Model file for the job. Use its own axes, mm. Face numbers are marked on the shaded views. Coordinates: 2 decimals unless noted, no trailing zeros. Order: outer loops, then holes, each group sorted by start corner. A loop starts at its lowest first (then second) coordinate and runs counter-clockwise, first axis right, second up. Notation, with made-up numbers: (-1.5, 16) -> (49.5, 16) arc R11 cw to (49.5, 22) -> close; hole circle Ø3 at (69, 8.25). An arc over 180 degrees is marked (long way). Use CSV: the item, a comma, the result in double quotes. Start each with the question number.
(1) Pin check, flat tips, straight feed: pin 1 Ø2 at (y, z) = (3, 116) entering from -X; pin 2 Ø1.9 at (x, z) = (0.5, 114.5) entering from +Y; pin 3 Ø1.6 at (y, z) = (1, 111) entering from +X. Stop position of each tip, or through.
(2) Cut at A-A on z = -25. Write the cut outline in (x, y).
(3) Probe L1, parallel to Y at x = 0, z = 99 (3 decimals); L2, parallel to Y at x = -13.5, z = -69.5; L3, parallel to Z at x = -13.5, y = -1.5. List the from-to ranges inside material, lowest first.
(4) Cut at B-B on z = -67. Write the cut outline in (x, y), plus the area to 3 significant figures.
(5) Pull direction Y, two halves, no side cores. Call the marked faces 1 and 2: pulls with the +Y half, pulls with the -Y half, needs draft (parallel to the pull), parting line crosses it, or undercut.
(6) Cut at C-C on z = 36. Write the cut outline in (x, y) (3 decimals).
```python
from build123d import *

# Parameters (mm, degrees)
PAD_DEPTH            = 25
PAD_DEPTH_BACK       = 25
PAD001_START         = 5
PAD001_DEPTH         = 115
PAD002_DEPTH         = 6
PAD002_DEPTH_BACK    = 6
POCKET_DEPTH         = 10.001
POCKET_DEPTH_BACK    = 10.001
POCKET001_DEPTH      = 120.001
PAD003_DEPTH         = 2
LINEARPATTERN_COUNT  = 2
LINEARPATTERN_PITCH  = 8
SKETCH006_W          = 15
SKETCH006_H          = 1
POCKET002_DEPTH      = 7
PAD004_DEPTH         = 6
PAD004_DEPTH_BACK    = 6
SKETCH008_W          = 3.8
SKETCH008_H          = 20
POCKET003_DEPTH      = 60.001
POCKET003_DEPTH_BACK = 60.001
POCKET004_DEPTH      = 10.001
POCKET004_DEPTH_BACK = 10.001
FILLET_R             = 10
FILLET001_R          = 10
FILLET002_R          = 5
FILLET003_R          = 10
FILLET004_R          = 1
FILLET005_R          = 1
SKETCH010_W          = 10
SKETCH010_H          = 30
POCKET005_DEPTH      = 60.001
POCKET005_DEPTH_BACK = 60.001
SKETCH011_W          = 10
SKETCH011_H          = 30
POCKET006_DEPTH      = 60.001
POCKET006_DEPTH_BACK = 60.001
FILLET006_R          = 10
CHAMFER_SIZE         = 1
CHAMFER001_SIZE      = 1


with BuildPart() as part:
    # Sketch → Pad (new body, two sides)
    with BuildSketch(Plane.YZ) as pad_sk:
        Polygon((10, -4.142136), (10, 4.142136), (4.142136, 10), (-4.142136, 10), (-10, 4.142136), (-10, -4.142136), (-4.142136, -10), (4.142136, -10), align=None)
        Polygon((2.5, 1.035534), (1.035534, 2.5), (-1.035534, 2.5), (-2.5, 1.035534), (-2.5, -1.035534), (-1.035534, -2.5), (1.035534, -2.5), (2.5, -1.035534), align=None, mode=Mode.SUBTRACT)
    extrude(amount=PAD_DEPTH)
    extrude(pad_sk.sketch, amount=-PAD_DEPTH_BACK)

    # Sketch001 → Pad001 (join)
    with BuildSketch(Plane.XY.offset(PAD001_START)):
        Polygon((4.5, -1.863961), (4.5, 1.863961), (1.863961, 4.5), (-1.863961, 4.5), (-4.5, 1.863961), (-4.5, -1.863961), (-1.863961, -4.5), (1.863961, -4.5), align=None)
        Polygon((1.575, -0.652386), (1.575, 0.652386), (0.652386, 1.575), (-0.652386, 1.575), (-1.575, 0.652386), (-1.575, -0.652386), (-0.652386, -1.575), (0.652386, -1.575), align=None, mode=Mode.SUBTRACT)
    extrude(amount=PAD001_DEPTH)

    # Sketch002 → Pad002 (join, two sides)
    with BuildSketch(Plane.XZ) as pad002_sk:
        Polygon((-25, 8), (25, 8), (25, 13), (10, 42), (10, 47), (13, 47), (13, 50), (-13, 50), (-13, 47), (-10, 47), (-10, 42), (-25, 13), align=None)
    extrude(amount=PAD002_DEPTH)
    extrude(pad002_sk.sketch, amount=-PAD002_DEPTH_BACK)

    # Sketch003 → Pocket (cut, two sides)
    with BuildSketch(Plane.XZ) as pocket_sk:
        with BuildLine():
            ThreePointArc((7, 8), (0, 15), (-7, 8))
            Line((-7, 8), (7, 8))
        make_face()
    extrude(amount=-POCKET_DEPTH, mode=Mode.SUBTRACT)
    extrude(pocket_sk.sketch, amount=POCKET_DEPTH_BACK, mode=Mode.SUBTRACT)

    # Sketch004 → Pocket001 (cut, through all)
    with BuildSketch(Plane.XY):
        Polygon((1.575, -0.652386), (1.575, 0.652386), (0.652386, 1.575), (-0.652386, 1.575), (-1.575, 0.652386), (-1.575, -0.652386), (-0.652386, -1.575), (0.652386, -1.575), align=None)
    extrude(amount=POCKET001_DEPTH, mode=Mode.SUBTRACT)

    # Sketch005 (on Face68 of Pocket001) → Pad003 (join)
    with BuildSketch(Plane(origin=(0, 0, 120), x_dir=(0, -1, 0), z_dir=(0, 0, 1))):
        Polygon((5.543277, -2.296101), (5.543277, 2.296101), (2.296101, 5.543277), (-2.296101, 5.543277), (-5.543277, 2.296101), (-5.543277, -2.296101), (-2.296101, -5.543277), (2.296101, -5.543277), align=None)
        Polygon((1.339392, -3.233578), (3.233578, -1.339392), (3.233578, 1.339392), (1.339392, 3.233578), (-1.339392, 3.233578), (-3.233578, 1.339392), (-3.233578, -1.339392), (-1.339392, -3.233578), align=None, mode=Mode.SUBTRACT)
    pad003 = extrude(amount=-PAD003_DEPTH)

    # LinearPattern: Pad003 ×2
    with Locations(*[(0, 0, -i * LINEARPATTERN_PITCH) for i in range(1, LINEARPATTERN_COUNT)]):
        add(pad003)

    # Sketch006 (on Face80 of LinearPattern) → Pocket002 (cut)
    with BuildSketch(Plane(origin=(0, 0, 120), x_dir=(0, -1, 0), z_dir=(0, 0, 1))):
        Rectangle(SKETCH006_W, SKETCH006_H)
    extrude(amount=-POCKET002_DEPTH, mode=Mode.SUBTRACT)

    # Sketch007 → Pad004 (join, two sides)
    with BuildSketch(Plane.XZ) as pad004_sk:
        Polygon((-25, -5), (25, -5), (25, -15), (60, -50), (60, -80), (-60, -80), (-60, -50), (-25, -15), align=None)
    extrude(amount=PAD004_DEPTH)
    extrude(pad004_sk.sketch, amount=-PAD004_DEPTH_BACK)

    # Sketch008 → Pocket003 (cut, two sides)
    with BuildSketch(Plane.YZ) as pocket003_sk:
        with Locations((0, -71)):
            Rectangle(SKETCH008_W, SKETCH008_H)
    extrude(amount=-POCKET003_DEPTH, mode=Mode.SUBTRACT)
    extrude(pocket003_sk.sketch, amount=POCKET003_DEPTH_BACK, mode=Mode.SUBTRACT)

    # Sketch009 → Pocket004 (cut, two sides)
    with BuildSketch(Plane.XZ) as pocket004_sk:
        Polygon((-5.142136, -8.142136), (5.142136, -8.142136), (45, -48), (45, -56), (-45, -56), (-45, -48), align=None)
    extrude(amount=-POCKET004_DEPTH, mode=Mode.SUBTRACT)
    extrude(pocket004_sk.sketch, amount=POCKET004_DEPTH_BACK, mode=Mode.SUBTRACT)

    # Fillet
    fillet_edges = [part.edges().sort_by_distance(p)[0] for p in [
        (25, 0, -15),
        (-25, 0, -15),
    ]]
    fillet(fillet_edges, radius=FILLET_R)

    # Fillet001
    fillet001_edges = [part.edges().sort_by_distance(p)[0] for p in [
        (-60, 0, -50),
        (60, 0, -50),
    ]]
    fillet(fillet001_edges, radius=FILLET001_R)

    # Fillet002
    fillet002_edges = [part.edges().sort_by_distance(p)[0] for p in [
        (-45, 0, -56),
        (-45, 0, -48),
        (45, 0, -48),
        (45, 0, -56),
    ]]
    fillet(fillet002_edges, radius=FILLET002_R)

    # Fillet003
    fillet003_edges = [part.edges().sort_by_distance(p)[0] for p in [
        (-25, 0, 13),
        (-10, 0, 42),
        (10, 0, 42),
        (25, 0, 13),
    ]]
    fillet(fillet003_edges, radius=FILLET003_R)

    # Fillet004
    fillet004_edges = [part.edges().sort_by_distance(p)[0] for p in [
        (10, 0, 47),
        (13, 0, 47),
        (13, 0, 50),
    ]]
    fillet(fillet004_edges, radius=FILLET004_R)

    # Fillet005
    fillet005_edges = [part.edges().sort_by_distance(p)[0] for p in [
        (-10, 0, 47),
        (-13, 0, 47),
        (-13, 0, 50),
    ]]
    fillet(fillet005_edges, radius=FILLET005_R)

    # Sketch010 → Pocket005 (cut, two sides)
    with BuildSketch(Plane.YZ) as pocket005_sk:
        with Locations((11, 0)):
            Rectangle(SKETCH010_W, SKETCH010_H)
    extrude(amount=-POCKET005_DEPTH, mode=Mode.SUBTRACT)
    extrude(pocket005_sk.sketch, amount=POCKET005_DEPTH_BACK, mode=Mode.SUBTRACT)

    # Sketch011 → Pocket006 (cut, two sides)
    with BuildSketch(Plane.YZ) as pocket006_sk:
        with Locations((-11, 0)):
            Rectangle(SKETCH011_W, SKETCH011_H)
    extrude(amount=-POCKET006_DEPTH, mode=Mode.SUBTRACT)
    extrude(pocket006_sk.sketch, amount=POCKET006_DEPTH_BACK, mode=Mode.SUBTRACT)

    # Fillet006
    fillet006_edges = [part.edges().sort_by_distance(p)[0] for p in [
        (60, -3.95, -80),
        (60, 3.95, -80),
        (-60, -3.95, -80),
        (-60, 3.95, -80),
    ]]
    fillet(fillet006_edges, radius=FILLET006_R)

    # Chamfer
    chamfer_edges = [part.edges().sort_by_distance(p)[0] for p in [
        (1.39805, 5.543277, 120),
        (3.919689, 3.919689, 120),
        (5.543277, 0, 120),
        (3.919689, -3.919689, 120),
        (1.39805, -5.543277, 120),
    ]]
    chamfer(chamfer_edges, length=CHAMFER_SIZE)

    # Chamfer001
    chamfer001_edges = [part.edges().sort_by_distance(p)[0] for p in [
        (-1.39805, 5.543277, 120),
        (-3.919689, 3.919689, 120),
        (-5.543277, 0, 120),
        (-3.919689, -3.919689, 120),
        (-1.39805, -5.543277, 120),
    ]]
    chamfer(chamfer001_edges, length=CHAMFER001_SIZE)


solid = part.part
```
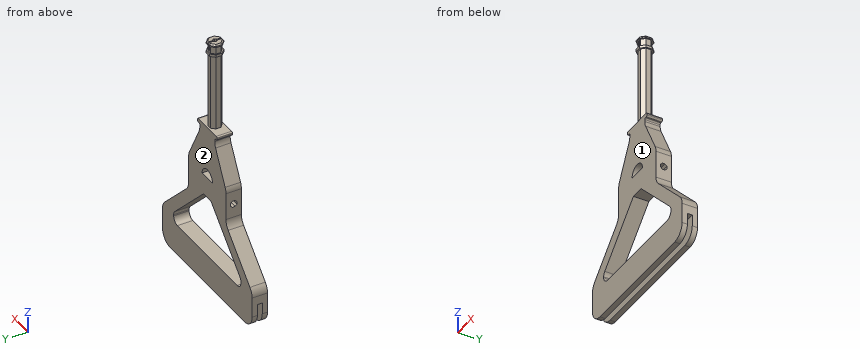
Outcome:
1,pin 1,"x = -4.36"
1,pin 2,"y = 4.5"
1,pin 3,"x = 5.54"
2,outline,"(-35, -6) -> (-22, -6) -> (-22, 6) -> (-35, 6) -> close; (22, -6) -> (35, -6) -> (35, 6) -> (22, 6) -> close"
3,L1,"-4.5 to -1.575, 1.575 to 4.5"
3,L2,"-6 to -1.9, 1.9 to 6"
3,L3,"-61 to -56, -16.5 to -2.04, 2.04 to 35.23"
4,outline,"(-60, -6) -> (60, -6) -> (60, -1.9) -> (-60, -1.9) -> close; (-60, 1.9) -> (60, 1.9) -> (60, 6) -> (-60, 6) -> close"
4,area,"984 mm2"
5,face 1,"pulls with the -Y half"
5,face 2,"pulls with the +Y half"
6,outline,"(-13.103, -6) -> (13.103, -6) -> (13.103, 6) -> (-13.103, 6) -> close; hole (-1.575, -0.652) -> (-0.652, -1.575) -> (0.652, -1.575) -> (1.575, -0.652) -> (1.575, 0.652) -> (0.652, 1.575) -> (-0.652, 1.575) -> (-1.575, 0.652) -> close"
